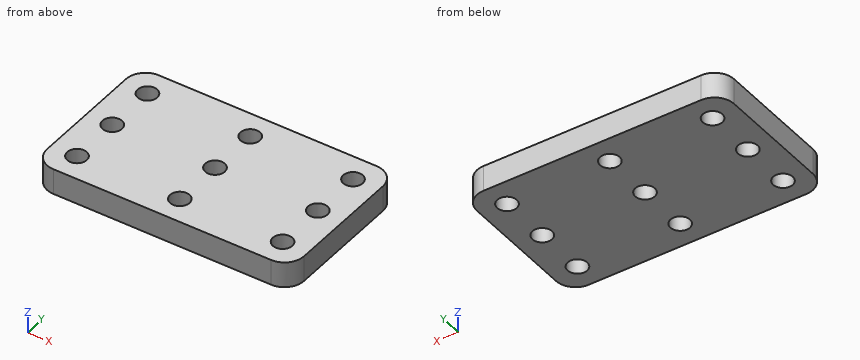
```python
from build123d import *

# Parameters (mm, degrees)
SKETCH1_W                     = 49.9999
SKETCH1_H                     = 29.99994
BOSS_EXTRUDE1_DEPTH           = 4.99999
SKETCH2_R                     = 1.905
CUT_EXTRUDE1_DEPTH            = 4.99999
LPATTERN1_COUNT               = 2
LPATTERN1_PITCH               = 9.99998
LPATTERN1_COL_COUNT           = 2
LPATTERN1_COL_PITCH           = 9.99998
LPATTERN2_COUNT               = 2
LPATTERN2_PITCH               = 19.99996
LPATTERN2_COPY_1_SKETCH_R     = 1.905
LPATTERN2_COPY_1_DEPTH        = 4.99999
LPATTERN2_COPY_2_SKETCH_R     = 1.905
LPATTERN2_COPY_2_DEPTH        = 4.99999
LPATTERN2_COL_COUNT           = 2
LPATTERN2_COL_PITCH           = 19.99996
LPATTERN2_COL_COPY_1_SKETCH_R = 1.905
LPATTERN2_COL_COPY_1_DEPTH    = 4.99999
LPATTERN2_COL_COPY_2_SKETCH_R = 1.905
LPATTERN2_COL_COPY_2_DEPTH    = 4.99999
FILLET1_R                     = 3.81


with BuildPart() as part:
    # Sketch1 → Boss-Extrude1 (new body)
    with BuildSketch(Plane.XY):
        Rectangle(SKETCH1_W, SKETCH1_H)
    extrude(amount=BOSS_EXTRUDE1_DEPTH)

    # Sketch2 → Cut-Extrude1 (cut)
    with BuildSketch(Plane.XY.offset(4.99999)):
        Circle(SKETCH2_R)
    cut_extrude1 = extrude(amount=-CUT_EXTRUDE1_DEPTH, mode=Mode.SUBTRACT)

    # LPattern1: Cut-Extrude1 ×2
    with Locations(*[(0, i * LPATTERN1_PITCH, 0) for i in range(1, LPATTERN1_COUNT)]):
        add(cut_extrude1, mode=Mode.SUBTRACT)

    # LPattern1 col: Cut-Extrude1 ×2
    with Locations(*[(0, -i * LPATTERN1_COL_PITCH, 0) for i in range(1, LPATTERN1_COL_COUNT)]):
        add(cut_extrude1, mode=Mode.SUBTRACT)

    # LPattern2: Cut-Extrude1 ×2
    with Locations(*[(-i * LPATTERN2_PITCH, 0, 0) for i in range(1, LPATTERN2_COUNT)]):
        add(cut_extrude1, mode=Mode.SUBTRACT)

    # LPattern2 copy 1 sketch → LPattern2 copy 1 (cut)
    with BuildSketch(Plane(origin=(-19.99996, 9.99998, 4.99999), x_dir=(1, 0, 0), z_dir=(0, 0, 1))):
        Circle(LPATTERN2_COPY_1_SKETCH_R)
    extrude(amount=-LPATTERN2_COPY_1_DEPTH, mode=Mode.SUBTRACT)

    # LPattern2 copy 2 sketch → LPattern2 copy 2 (cut)
    with BuildSketch(Plane(origin=(-19.99996, -9.99998, 4.99999), x_dir=(1, 0, 0), z_dir=(0, 0, 1))):
        Circle(LPATTERN2_COPY_2_SKETCH_R)
    extrude(amount=-LPATTERN2_COPY_2_DEPTH, mode=Mode.SUBTRACT)

    # LPattern2 col: Cut-Extrude1 ×2
    with Locations(*[(i * LPATTERN2_COL_PITCH, 0, 0) for i in range(1, LPATTERN2_COL_COUNT)]):
        add(cut_extrude1, mode=Mode.SUBTRACT)

    # LPattern2 col copy 1 sketch → LPattern2 col copy 1 (cut)
    with BuildSketch(Plane(origin=(19.99996, 9.99998, 4.99999), x_dir=(1, 0, 0), z_dir=(0, 0, 1))):
        Circle(LPATTERN2_COL_COPY_1_SKETCH_R)
    extrude(amount=-LPATTERN2_COL_COPY_1_DEPTH, mode=Mode.SUBTRACT)

    # LPattern2 col copy 2 sketch → LPattern2 col copy 2 (cut)
    with BuildSketch(Plane(origin=(19.99996, -9.99998, 4.99999), x_dir=(1, 0, 0), z_dir=(0, 0, 1))):
        Circle(LPATTERN2_COL_COPY_2_SKETCH_R)
    extrude(amount=-LPATTERN2_COL_COPY_2_DEPTH, mode=Mode.SUBTRACT)

    # Fillet1
    fillet1_edges = [part.edges().sort_by_distance(p)[0] for p in [
        (24.99995, -14.99997, 2.499995),
        (-24.99995, -14.99997, 2.499995),
        (-24.99995, 14.99997, 2.499995),
        (24.99995, 14.99997, 2.499995),
    ]]
    fillet(fillet1_edges, radius=FILLET1_R)


solid = part.part
```
Can you work these out from the model? Positions are in its coordinate system, mm. Round coordinates to 2 decimals unless told otherwise and drop trailing zeros. Order: outer loops, then holes, each group sorted by start corner. A loop starts at its lowest first (then second) coordinate and runs counter-clockwise, first axis right, second up. Notation, with made-up numbers: (48.5, -35) -> (73.5, -35) arc R26 ccw to (73.5, -10) -> close; hole circle Ø2 at (-14.75, 24.5). An arc over 180 degrees is marked (long way). Return JSON: item names as keys, results as strings. Group by question number.
1. Will these pins go through, and if not, where does the flat tip stop? pin 1 (2 mm diameter, centred on x = 16.5, y = 5.5, fed in from -Z); pin 2 (3.5 mm diameter, centred on x = -20, y = 10, fed in from -Z).
2. I need wall thicknesses on line 1 (X direction, y = 10, z = 3.85) (3 decimals); line 2 (Y direction, x = 0, z = 4.8) (3 decimals); line 3 (X direction, y = -11, z = 4.05). Which ranges of each line are inside material? Lowest first, please. Write a range as [from, to].
3. If we section it at C-C, the plane z = 3.9: Count the separate pieces of the cut face and the enclosed holes in it, then the cut area to 3 significant figures.
4. If we section it at A-A, the plane y = 0: Write out the boundary of the cut face in (x, z) (3 decimals), then the cut area to 3 significant figures.
5. If we section it at B-B, the plane x = -20: Write out the boundary of the cut face in (y, z) (3 decimals).
Output values:
{
 "1": {"pin 1": "z = 0", "pin 2": "through"},
 "2": {"line 1": "[-25, -21.905], [-18.095, -1.905], [1.905, 18.095], [21.905, 25]", "line 2": "[-15, -11.905], [-8.095, -1.905], [1.905, 8.095], [11.905, 15]", "line 3": "[-25, -21.62], [-18.38, -1.62], [1.62, 18.38], [21.62, 25]"},
 "3": {"separate pieces": "1", "enclosed holes": "9", "area": "1,380 mm²"},
 "4": {"outline": "(-25, 0) -> (-21.905, 0) -> (-21.905, 5) -> (-25, 5) -> close; (-18.095, 0) -> (-1.905, 0) -> (-1.905, 5) -> (-18.095, 5) -> close; (1.905, 0) -> (18.095, 0) -> (18.095, 5) -> (1.905, 5) -> close; (21.905, 0) -> (25, 0) -> (25, 5) -> (21.905, 5) -> close", "area": "193 mm²"},
 "5": {"outline": "(-15, 0) -> (-11.905, 0) -> (-11.905, 5) -> (-15, 5) -> close; (-8.095, 0) -> (-1.905, 0) -> (-1.905, 5) -> (-8.095, 5) -> close; (1.905, 0) -> (8.095, 0) -> (8.095, 5) -> (1.905, 5) -> close; (11.905, 0) -> (15, 0) -> (15, 5) -> (11.905, 5) -> close"}
}
